```python
from build123d import *

# Parameters (mm, degrees)
SKETCH1_W           = 68.6
SKETCH1_H           = 53.3
BOSS_EXTRUDE1_DEPTH = 1.6
SKETCH2_W           = 15
SKETCH2_H           = 12
SKETCH2_W_2         = 13
SKETCH2_H_2         = 8.9
BOSS_EXTRUDE2_DEPTH = 10.9
SKETCH3_R           = 1.75
CUT_EXTRUDE1_DEPTH  = 2.6
SKETCH4_R           = 7.5
BOSS_EXTRUDE3_DEPTH = 14


with BuildPart() as part:
    # Sketch1 → Boss-Extrude1 (new body)
    with BuildSketch(Plane.XY):
        Rectangle(SKETCH1_W, SKETCH1_H)
    extrude(amount=BOSS_EXTRUDE1_DEPTH)

    # Sketch2 → Boss-Extrude2 (add)
    with BuildSketch(Plane.XY.offset(1.6)):
        with Locations((-33, 11.05)):
            Rectangle(SKETCH2_W, SKETCH2_H)
        with Locations((-29.6, -18.9)):
            Rectangle(SKETCH2_W_2, SKETCH2_H_2)
    extrude(amount=BOSS_EXTRUDE2_DEPTH)

    # Sketch3 → Cut-Extrude1 (cut, through all)
    with BuildSketch(Plane.XY.offset(1.6)):
        with Locations((-19, 24.05)):
            Circle(SKETCH3_R)
        with Locations((-20.3, -24.15)):
            Circle(SKETCH3_R)
        with Locations((31.8, -19.05)):
            Circle(SKETCH3_R)
        with Locations((31.8, 8.85)):
            Circle(SKETCH3_R)
    extrude(amount=-CUT_EXTRUDE1_DEPTH, mode=Mode.SUBTRACT)

    # Sketch4 → Boss-Extrude3 (add)
    with BuildSketch(Plane.XY.offset(1.6)):
        Circle(SKETCH4_R)
    extrude(amount=BOSS_EXTRUDE3_DEPTH)


solid = part.part
```
Input: part model. Units: mm. Frame: model coordinates. A direction names the side the tool comes from. Coordinates: 2 decimals unless noted, no trailing zeros. Order: outer loops, then holes, each group sorted by start corner. A loop starts at its lowest first (then second) coordinate and runs counter-clockwise, first axis right, second up. Notation, with made-up numbers: (43, 12) - (80, 12) arc R15 cw to (80, 20) - close; hole circle Ø5 at (-21.5, 3.25). An arc over 180 degrees is marked (long way). Return JSON: item names as keys, results as strings.
Q1. Ray query, probe 1 along Y at (x, z) = (31.8, 1.25); probe 2 along Y at (x, z) = (-20, 1); probe 3 along Y at (x, z) = (-32.5, 4.25). Return the intervals inside material, ascending.
The answers:
{"probe 1": "y = -26.65 to -20.8, -17.3 to 7.1, 10.6 to 26.65", "probe 2": "y = -26.65 to -25.87, -22.43 to 22.61, 25.49 to 26.65", "probe 3": "y = -23.35 to -14.45, 5.05 to 17.05"}
Q2. Cut plane A-A (y = -19.05). Return loops of the section in (x, z), then the cut area to 3 significant figures.
The answers:
{"outline": "(-36.1, 1.6) - (-34.3, 1.6) - (-34.3, 0) - (30.05, 0) - (30.05, 1.6) - (-23.1, 1.6) - (-23.1, 12.5) - (-36.1, 12.5) - close; (33.55, 0) - (34.3, 0) - (34.3, 1.6) - (33.55, 1.6) - close", "area": "246 mm2"}
Q3. Cut plane D-D (x = -19.5). Return loops of the section in (y, z).
The answers:
{"outline": "(-26.65, 0) - (-25.71, 0) - (-25.71, 1.6) - (-26.65, 1.6) - close; (-22.59, 0) - (22.37, 0) - (22.37, 1.6) - (-22.59, 1.6) - close; (25.73, 0) - (26.65, 0) - (26.65, 1.6) - (25.73, 1.6) - close"}
Q4. First-contact query: pin 1 (8 mm diameter, centred on y = -6.5, z = 8, fed in from +X); pin 2 (7 mm diameter, centred on y = -17, z = 6, fed in from -X); pin 3 (3 mm diameter, centred on x = -26, z = 7, fed in from +Y); pin 4 (2 mm diameter, centred on x = 31.8, y = 8.85, fed in from -Z). Flat tips, straight axial feed; report the tip coordinate or a pass-through.
The answers:
{"pin 1": "stops at x = 7.07", "pin 2": "stops at x = -36.1", "pin 3": "stops at y = 17.05", "pin 4": "passes through"}
Q5. Draft query along Y for faces 6 (the cylindrical face through (-7.493, 0.33, 8.502)), 7 (the cylindrical face through (-20.29, 25.23, 0.81)), 8 (the flat face through (-36.1, -19, 7)). Return one class per face: +Y half, -Y half, draft (parallel to the pull), parting line (faces both ways), or undercut.
The answers:
{"face 6": "parting line", "face 7": "undercut", "face 8": "draft"}
Q6. Cut plane C-C (y = 0). Return loops of the section in (x, z).
The answers:
{"outline": "(-34.3, 0) - (34.3, 0) - (34.3, 1.6) - (7.5, 1.6) - (7.5, 15.6) - (-7.5, 15.6) - (-7.5, 1.6) - (-34.3, 1.6) - close"}
Q7. Access query for faces 1 (the flat face through (-35, -19, 1.6)), 2 (the flat face through (-33, 17.05, 7)), 3 (the flat face through (-33, 5.05, 7)), 4 (the flat face through (-33, 11, 12.5)), 5 (the flat face through (-23.1, -19, 7)). Directions: +Z, -Z, +X, -X, +Y, -Y. A direction counts if a zero-diameter tool reaches every point of the face in a straight line with its end or side. Return the directions, or none.
The answers:
{"face 1": "-Z, -X, +Y, -Y", "face 2": "+Z, +X, -X, +Y", "face 3": "+Z, -X", "face 4": "+Z, -X, +Y, -Y", "face 5": "+Z, +X, +Y, -Y"}
Q8. Cut plane B-B (z = 11.5). Return loops of the section in (x, y), then the cut area to 3 significant figures.
The answers:
{"outline": "(-40.5, 5.05) - (-25.5, 5.05) - (-25.5, 17.05) - (-40.5, 17.05) - close; (-36.1, -23.35) - (-23.1, -23.35) - (-23.1, -14.45) - (-36.1, -14.45) - close; circle Ø15 at (0, 0)", "area": "472 mm2"}
